Check sheet for the modelled part. Datum: model origin and axes. Units: mm. A direction names the side the tool comes from. Give positions to 0.01 mm unless a question says otherwise; leave off trailing zeros. Order: outer loops, then holes, each group sorted by start corner. A loop starts at its lowest first (then second) coordinate and runs counter-clockwise, first axis right, second up. Notation, with made-up numbers: M 74,21.25 L 84,21.25 A18 cw 84,45.25 Z; hole C 52,42.5 d3. An arc over 180 degrees is marked long. Answer in a Markdown table with one row per item. Add a question column.
from build123d import *

# Parameters (mm, degrees)
SKETCH1_R           = 1
SKETCH1_W           = 13
SKETCH1_H           = 24
BOSS_EXTRUDE1_DEPTH = 3


with BuildPart() as part:
    # Sketch1 → Boss-Extrude1 (new body)
    with BuildSketch(Plane.XY):
        Polygon((30.8, 14), (33.8, 14), (33.8, 10), (30.8, 10), (30.8, 6), (33.8, 6), (33.8, 2), (30.8, 2), (30.8, -2), (33.8, -2), (33.8, -6), (30.8, -6), (30.8, -10), (33.8, -10), (33.8, -14), (30.8, -14), (30.8, -16), (-8.5, -16), (-8.5, 16), (30.8, 16), align=None)
        with Locations((0, 13.625)):
            Circle(SKETCH1_R, mode=Mode.SUBTRACT)
        with Locations(Location((0, -13.625, 0), (0, 0, 180))):
            Circle(SKETCH1_R, mode=Mode.SUBTRACT)
        Rectangle(SKETCH1_W, SKETCH1_H, mode=Mode.SUBTRACT)
    extrude(amount=BOSS_EXTRUDE1_DEPTH)


solid = part.part
Q1. Cross-section at D-D (z = 1.2). Record the boundary of the cut face in (x, y) (3 decimals).
Q2. Tool access check on faces 1 (the flat face through (0, -12, 1)), 2 (the flat face through (30.8, -15, 1)), 3 (the flat face through (11, 16, 1)), 4 (the flat face through (30.8, 8, 1)). Record the directions out of +Z, -Z, +X, -X, +Y, -Y that give a thin tool (end or side, any length) a straight path to the whole face; none if there is none.
Q3. Cross-section at C-C (x = 0). Record the boundary of the cut face in (y, z) (3 decimals).
Q4. Thickness scan on probe 1 along Y at (x, z) = (0, 1.35) (3 decimals); probe 2 along Y at (x, z) = (32.5, 1.4); probe 3 along X at (y, z) = (-7, 1.65). Record the ranges inside material, lowest first.
Q5. Cross-section at B-B (x = 4.5). Record the boundary of the cut face in (y, z), and give its area (3 significant figures).
Q6. Draft check along Y on faces 5 (the flat face through (11, -16, 1)), 6 (the flat face through (33.8, 4, 1)), 7 (the flat face through (30.8, -8, 1)). Enter one of: pulls with the +Y half, pulls with the -Y half, needs draft (parallel to the pull), parting line crosses it, or undercut.
Q7. Cross-section at A-A (y = 8). Record the boundary of the cut face in (x, z).
Q8. Go/stop test with flat-tipped pins: pin 1 (1.5 mm diameter, centred on x = 33, z = 2, fed in from +Y); pin 2 (1.5 mm diameter, centred on y = 0, z = 2, fed in from +X). Record where each tip stops, or that it passes through.
Values follow:
| question | item | result |
|---|---|---|
| 1 | outline | M -8.5,-16 L 30.8,-16 L 30.8,-14 L 33.8,-14 L 33.8,-10 L 30.8,-10 L 30.8,-6 L 33.8,-6 L 33.8,-2 L 30.8,-2 L 30.8,2 L 33.8,2 L 33.8,6 L 30.8,6 L 30.8,10 L 33.8,10 L 33.8,14 L 30.8,14 L 30.8,16 L -8.5,16 Z; hole M -6.5,-12 L 6.5,-12 L 6.5,12 L -6.5,12 Z; hole C 0,-13.625 d2; hole C 0,13.625 d2 |
| 2 | face 1 | +Z, -Z |
| 2 | face 2 | +Z, -Z, +X, -Y |
| 2 | face 3 | +Z, -Z, +X, -X, +Y |
| 2 | face 4 | +Z, -Z, +X |
| 3 | outline | M -16,0 L -14.625,0 L -14.625,3 L -16,3 Z; M -12.625,0 L -12,0 L -12,3 L -12.625,3 Z; M 12,0 L 12.625,0 L 12.625,3 L 12,3 Z; M 14.625,0 L 16,0 L 16,3 L 14.625,3 Z |
| 4 | probe 1 | -16 to -14.625, -12.625 to -12, 12 to 12.625, 14.625 to 16 |
| 4 | probe 2 | -14 to -10, -6 to -2, 2 to 6, 10 to 14 |
| 4 | probe 3 | -8.5 to -6.5, 6.5 to 30.8 |
| 5 | outline | M -16,0 L -12,0 L -12,3 L -16,3 Z; M 12,0 L 16,0 L 16,3 L 12,3 Z |
| 5 | area | 24.0 mm² |
| 6 | face 5 | pulls with the -Y half |
| 6 | face 6 | needs draft |
| 6 | face 7 | undercut |
| 7 | outline | M -8.5,0 L -6.5,0 L -6.5,3 L -8.5,3 Z; M 6.5,0 L 30.8,0 L 30.8,3 L 6.5,3 Z |
| 8 | pin 1 | y = 14 |
| 8 | pin 2 | x = 30.8 |
